Autodesk Inventor part; units mm, degrees
ref_plane "YZ Plane" through (0, 0, 0) normal (1, 0, 0) x (0, 1, 0)
ref_plane "XZ Plane" through (0, 0, 0) normal (0, 1, 0) x (-1, 0, 0)
ref_plane "XY Plane" through (0, 0, 0) normal (0, 0, 1) x (1, 0, 0)
sketch "Skizze1" plane through (0, 0, 0) normal (0, 0, 1) x (1, 0, 0)
  circle A0 centre (0, 0) radius 4 construction
  circle A1 centre (-25, 0) radius 4 construction
  line L0 (-25, 0) -> (0, 0) construction
  line L1 (-29, 0) -> (-29, -4)
  line L2 (-29, -4) -> (0, -4)
  line L3 (0, 4) -> (-25, 4)
  arc A2 (-25, 4) -> (-29, 0) centre (-25, 0) ccw
  arc A3 (0, -4) -> (0, 4) centre (0, 0) ccw
  dimension "d0" = 8
  dimension "d1" = 25
extrude "Extrusion1" add sketch "Skizze1" along normal blind 3
sketch "Skizze2" plane through (0, 0, 0) normal (0, 0, -1) x (-1, 0, 0)
  arc A0 (29, 0) -> (25, 4) centre (25, 0) ccw
  line L0 (0, 4) -> (25, 4)
  arc A1 (0, 4) -> (0, -4) centre (0, 0) ccw
  line L1 (29, -4) -> (0, -4)
  line L2 (6, 4) -> (19, 4)
  line L3 (19, 4) -> (19, -4)
  line L4 (19, -4) -> (6, -4)
  line L5 (6, -4) -> (6, 4)
  dimension "d4" = 4
  dimension "d5" = 6
  dimension "d6" = 6
extrude "Extrusion2" add sketch "Skizze2" along normal blind 9.5 contours L0 L3 L1 L5
sketch "Skizze3" plane through (0, 0, 0) normal (0, 0, -1) x (-1, 0, 0)
  line L0 (6, -4) -> (6, 4)
  line L1 (0, 4) -> (6, 4)
  arc A0 (0, 4) -> (0, -4) centre (0, 0) ccw
  line L2 (6, -4) -> (0, -4)
extrude "Extrusion3" add sketch "Skizze3" along normal blind 3
sketch "Skizze4" plane through (0, 0, 3) normal (0, 0, 1) x (1, 0, 0)
  line L0 (-6, 4) -> (-6, -4)
  line L1 (-6, 4) -> (0, 4)
  arc A0 (0, -4) -> (0, 4) centre (0, 0) ccw
  line L2 (0, -4) -> (-6, -4)
extrude "Extrusion4" cut sketch "Skizze4" against normal blind 3
mirror "Spiegeln1" about plane through (-12.5, 0, -9.5) normal (0, 0, -1)
sketch "Skizze5" plane through (0, 0, 0) normal (0, 0, -1) x (-1, 0, 0)
  line L0 (19, 4) -> (19, -4)
  line L1 (19, 4) -> (25, 4)
  line L2 (19, 4) -> (13.3983, -4)
  line L3 (13.3983, -4) -> (19, -4)
  point P0 (0, 0)
  dimension "d13" = 35
extrude "Extrusion5" cut sketch "Skizze5" along normal up to surface (19 mm away)
sketch "Skizze6" plane through (0, 0, 3) normal (0, 0, 1) x (1, 0, 0)
  arc A0 (-25, 4) -> (-29, 0) centre (-25, 0) ccw
  point P0 (0, 0)
hole "Bohrung1" at (-25, 0, 3) direction (0, 0, -1) diameter 3 end through all
hole "Bohrung2" at (0, 0, 3) direction (0, 0, -1) diameter 3 end through all
sketch "Skizze7" plane through (-6, -4, 3) normal (1, 0, 0) x (0, 0, -1)
  line L0 (0, 0) -> (0, 8)
  line L1 (3, 0) -> (0, 0)
  line L2 (3, 0) -> (3, 8)
  line L3 (0, 8) -> (3, 8)
  line L4 (22, 0) -> (25, 0)
  line L5 (25, 0) -> (25, 8)
  line L6 (25, 8) -> (22, 8)
  line L7 (22, 0) -> (22, 8)
  line L8 (22, 0) -> (25, 0)
  point P0 (3, 4)
extrude "Extrusion6" add sketch "Skizze7" along normal blind 2
chamfer "Fase1" distance 2 angle 45 1 edges at (-6, -4, -9.5)
sketch "Skizze8" plane through (-25, 4, 3) normal (0, 1, 0) x (1, 0, 0)
  line L0 (17, 19) -> (25, 19)
  line L1 (17, 6) -> (17, 19)
  line L2 (25, 6) -> (17, 6)
  line L3 (25, 6) -> (25, 3)
  line L4 (25, 3) -> (21, 3)
  line L5 (21, 0) -> (21, 3)
  line L6 (-4, 0) -> (21, 0)
  line L7 (-4, 3) -> (-4, 0)
  line L8 (-4, 3) -> (11.6017, 3)
  line L9 (11.6017, 3) -> (11.6017, 22)
  line L10 (11.6017, 22) -> (-4, 22)
  line L11 (-4, 22) -> (-4, 25)
  line L12 (-4, 25) -> (21, 25)
  line L13 (21, 22) -> (21, 25)
  line L14 (25, 22) -> (21, 22)
  line L15 (25, 19) -> (25, 22)
  line L16 (17, 19) -> (11.6017, 19)
  line L17 (17, 6) -> (11.6017, 6)
  point P0 (14.3008, 19)
  point P1 (14.3008, 6)
hole "Bohrung3" at (-10.6992, 4, -16) at (-10.6992, 4, -3) direction (0, -1, 0) diameter 2.5 end through all countersink diameter 4 countersink angle 90
sketch "Skizze9" plane through (0, 0, 0) normal (0, 0, 1) x (1, 0, 0)
  line L0 (-4, 4) -> (-4, -4)
  line L1 (0, -4) -> (-4, -4)
  arc A0 (0, -4) -> (0, 4) centre (0, 0) ccw
  line L2 (-4, 4) -> (0, 4)
  circle A1 centre (0, 0) radius 1.5
  circle A2 centre (0, 0) radius 4
equation "\"d0\" = Finger_diameter"
equation "\"d1\" = FingerLaenge_B"
equation "\"d2\" = FingerWall"
equation "\"d5\" = 1.5 * d4"
equation "\"d6\" = d5"
equation "\"d7\" = -0.5 * FingerWall + 0.5 * Finger_width"
equation "\"d9\" = FingerWall"
equation "\"d11\" = FingerWall"
equation "\"d29\" = bearingHole"
equation "\"FingerLaenge_B\" = 25"
equation "\"Hebel_B\" = 25"
equation "\"Finger_width\" = 22"
equation "\"Finger_diameter\" = 8"
equation "\"FingerWall\" = 3"
equation "\"Hebel_basis_2\" = 15"
equation "\"Join_width\" = 3"
equation "\"bearingHole\" = 3"
equation "\"bearingWall\" = 4"
equation "\"support_D\" = 0.25"
properties part number "FingerPartB"
Build history of the part. All positions in model axes, mm. A direction names the side the tool comes from. Coordinates: 2 decimals unless noted, no trailing zeros. Order: outer loops, then holes, each group sorted by start corner. A loop starts at its lowest first (then second) coordinate and runs counter-clockwise, first axis right, second up. Notation, with made-up numbers: (70.5, 86.25) - (84.5, 86.25) arc R27 cw to (84.5, 109.25) - close; hole circle Ø9 at (-33.75, 51.5). An arc over 180 degrees is marked (long way). Put each result on its own line as item: value.
1. Tool access for faces 1 (the face through (-9.59, -0.43, -2.42)), 2 (the face through (-2, 0, -19)), 3 (the face through (-23, 0, -19)), 4 (the face through (-2, 0, 0)), 5 (the face through (-7, -3, -9)): list every direction of +Z, -Z, +X, -X, +Y, -Y with a clear straight run to the whole face (end or side of a thin tool).
Answer sheet:
face 1: +Y, -Y
face 2: -Z, +X, +Y, -Y
face 3: -X, -Y
face 4: +Z, +X, +Y, -Y
face 5: +X, -Y
2. Saw through at D-D (y = -3). Write the cut outline in (x, z).
Answer sheet:
outline: (-29, -22) - (-4, -22) - (-4, -19) - (2.65, -19) - (2.65, -16) - (-7, -16) - (-7, -3) - (2.65, -3) - (2.65, 0) - (-4, 0) - (-4, 3) - (-29, 3) - (-29, 0) - (-14.1, 0) - (-14.1, -19) - (-29, -19) - close; hole circle Ø2.5 at (-10.7, -16); hole circle Ø2.5 at (-10.7, -3)
3. Probe line 1 along Z through (x, y) = (-26.5, 0.75); line 2 along Z through (x, y) = (2.5, 2); line 3 along X through (y, z) = (0, 2.25). List the from-to ranges inside material, lowest first. Write a range as [from, to].
Answer sheet:
line 1: z = [-22, -19], [0, 3]
line 2: z = [-19, -16], [-3, 0]
line 3: x = [-29, -26.5], [-23.5, -4]
4. Drop flat-ended pins along their axis: P1, Ø8, axis at x = -12.5, z = -2.5, coming from the +Y side; P2, Ø0.9, axis at y = 0, z = 1, coming from the +X side; P3, Ø4, axis at x = -1.5, y = 0.5, coming from the +Z side; P4, Ø1.5, axis at y = -1.5, z = -5.5, coming from the -X side. Give the stop position or say it passes through.
Answer sheet:
P1: stops at y = 4
P2: stops at x = -4
P3: stops at z = 0
P4: stops at x = -15.67
5. Pull direction Z, two halves, no side cores. Call faces 6 (the face through (-0.07, 1.5, -17.52)), 7 (the face through (-16, 0, -22)), 8 (the face through (-9.48, -0.43, -16.27)): pulls with the +Z half, pulls with the -Z half, needs draft (parallel to the pull), parting line crosses it, or undercut.
Answer sheet:
face 6: needs draft
face 7: pulls with the -Z half
face 8: undercut
6. Saw through at A-A (x = -5.5). Write the cut outline in (y, z).
Answer sheet:
outline: (-4, -22) - (4, -22) - (4, -16) - (-4, -16) - close; (-4, -3) - (4, -3) - (4, 3) - (-4, 3) - close
7. Saw through at B-B (y = 1). Give the number of separate pieces and of enclosed holes in the cut face, and give its area (3 significant figures).
Answer sheet:
separate pieces: 5
enclosed holes: 2
area: 379 mm^2
8. Saw through at C-C (x = -1). Write the cut outline in (y, z).
Answer sheet:
outline: (-4, -19) - (-1.12, -19) - (-1.12, -16) - (-4, -16) - close; (-4, -3) - (-1.12, -3) - (-1.12, 0) - (-4, 0) - close; (1.12, -19) - (4, -19) - (4, -16) - (1.12, -16) - close; (1.12, -3) - (4, -3) - (4, 0) - (1.12, 0) - close
